```python
from build123d import *

# Parameters (mm, degrees)
SKETCH1_R           = 20
SKETCH1_R_2         = 17.5
BOSS_EXTRUDE1_DEPTH = 20
SKETCH2_R           = 32
SKETCH2_R_2         = 20
BOSS_EXTRUDE2_DEPTH = 3
SKETCH4_W           = 2.75
SKETCH4_H           = 3
CIRPATTERN1_COUNT   = 3
CHAMFER1_SIZE       = 1
SKETCH5_R           = 21.1
SKETCH5_R_2         = 18.5
CUT_EXTRUDE1_DEPTH  = 1.6
FILLET1_R           = 0.25
FILLET2_R           = 0.1
FILLET3_R           = 1


with BuildPart() as part:
    # Sketch1 → Boss-Extrude1 (new body, symmetric)
    with BuildSketch(Plane.XY):
        Circle(SKETCH1_R)
        Circle(SKETCH1_R_2, mode=Mode.SUBTRACT)
    extrude(amount=BOSS_EXTRUDE1_DEPTH, both=True)

    # Chamfer1
    chamfer1_edges = [part.edges().sort_by_distance(p)[0] for p in [
        (-17.5, 0, -20),
    ]]
    chamfer(chamfer1_edges, length=CHAMFER1_SIZE)


with BuildPart() as body_2:
    # Sketch2 → Boss-Extrude2 (new body)
    with BuildSketch(Plane.XY.offset(20)):
        Circle(SKETCH2_R)
        Circle(SKETCH2_R_2, mode=Mode.SUBTRACT)
    extrude(amount=-BOSS_EXTRUDE2_DEPTH)

    # Sketch4 → M5 Clearance Hole1 (revolve, cut)
    with BuildSketch(Plane(origin=(0, 26, 17), x_dir=(0, 1, 0), z_dir=(1, 0, 0))):
        with Locations((1.375, 1.5)):
            Rectangle(SKETCH4_W, SKETCH4_H)
    m5_clearance_hole1 = revolve(axis=Axis((0, 26, 10.65), (0, 0, 1)), mode=Mode.SUBTRACT)

    # CirPattern1: M5 Clearance Hole1 ×3 about axis
    cirpattern1_axis = Axis((0, 0, 0), (0, 0, 1))
    for i in range(1, CIRPATTERN1_COUNT):
        add(m5_clearance_hole1.rotate(cirpattern1_axis, i * 360 / CIRPATTERN1_COUNT), mode=Mode.SUBTRACT)


with BuildPart() as part_1:
    add(part.part)

    # Combine1: union body 2
    add(body_2.part)

    # Sketch5 → Cut-Extrude1 (cut)
    with BuildSketch(Plane.XY.offset(20)):
        Circle(SKETCH5_R)
        Circle(SKETCH5_R_2, mode=Mode.SUBTRACT)
    extrude(amount=-CUT_EXTRUDE1_DEPTH, mode=Mode.SUBTRACT)

    # Fillet1
    fillet1_edges = [part_1.edges().sort_by_distance(p)[0] for p in [
        (-21.1, 0, 18.4),
        (-18.5, 0, 18.4),
    ]]
    fillet(fillet1_edges, radius=FILLET1_R)

    # Fillet2
    fillet2_edges = [part_1.edges().sort_by_distance(p)[0] for p in [
        (-21.1, 0, 20),
        (-18.5, 0, 20),
    ]]
    fillet(fillet2_edges, radius=FILLET2_R)

    # Fillet3
    fillet3_edges = [part_1.edges().sort_by_distance(p)[0] for p in [
        (-20, 0, 17),
    ]]
    fillet(fillet3_edges, radius=FILLET3_R)


solid = part_1.part
```
The listing builds one solid part. Answer for the finished solid, in the listing's coordinates (mm). A direction names the side the tool comes from. Give positions to 0.01 mm unless a question says otherwise; leave off trailing zeros. Order: outer loops, then holes, each group sorted by start corner. A loop starts at its lowest first (then second) coordinate and runs counter-clockwise, first axis right, second up.
1) Find section A-A on x = -22. Write down the section's boundary in (y, z), then the cut area to 3 significant figures.
Reported:
outline: (-23.24, 17) - (-15.7, 17) - (-15.7, 20) - (-23.24, 20) - close; (-10.3, 17) - (23.24, 17) - (23.24, 20) - (-10.3, 20) - close
area: 123 mm2
2) For faces 1 (the face through (20.126, 6.338, 19.284)), 2 (the face through (-4.336, -19.524, -1.748)), 3 (the face through (-19.832, -13.596, 18.521)), determine the directions among +Z, -Z, +X, -X, +Y, -Y from which every point of the face is accessible in a straight line to the end or side of a thin tool.
Reported:
face 1: +Z
face 2: -Z
face 3: +Z, -Z
3) Determine the mould class of faces 4 (the face through (-6.94, -31.24, 18.52)), 5 (the face through (-19, 3, 18.4)), 6 (the face through (6, -18, -20)) for opening direction Y: pulls with the +Y half, pulls with the -Y half, needs draft (parallel to the pull), parting line crosses it, or undercut.
Reported:
face 4: parting line crosses it
face 5: undercut
face 6: needs draft
4) Find section B-B on z = -7. Write down the section's boundary in (x, y), then the cut area to 3 significant figures.
Reported:
outline: circle Ø40 at (0, 0); hole circle Ø35 at (0, 0)
area: 295 mm2
5) Find section D-D on x = 0. Give the number of separate pieces and of enclosed holes in the cut face, then the cut area to 3 significant figures.
Reported:
separate pieces: 3
enclosed holes: 0
area: 247 mm2
6) Find section C-C on y = 26. Write down the section's boundary in (x, z), then the cut area to 3 significant figures.
Reported:
outline: (-18.65, 17) - (-2.75, 17) - (-2.75, 20) - (-18.65, 20) - close; (2.75, 17) - (18.65, 17) - (18.65, 20) - (2.75, 20) - close
area: 95.4 mm2
7) Consider line 1 along X through (y, z) = (-0.5, 11.5); line 2 along Z through (x, y) = (-5, -23); line 3 along X through (y, z) = (-13, 18.15). Determine where each line is inside the solid, lowest interval first.
Reported:
line 1: x = -19.99 to -17.49, 17.49 to 19.99
line 2: z = 17 to 20
line 3: x = -29.24 to -25.27, -19.77 to -11.72, 11.72 to 19.77, 25.27 to 29.24
8) Given P1, Ø3, axis at x = -6.5, z = 4.5, coming from the +Y side; P2, Ø8, axis at y = 14.5, z = 13.5, coming from the -X side; P3, Ø5, axis at x = 0, y = 26, coming from the +Z side (3 decimals); P4, Ø5, axis at x = 12, z = 7.5, coming from the +Y side, each flat-ended and moving along its own axis, determine where each tip first touches the part or whether it passes through.
Reported:
P1: stops at y = 19.36
P2: stops at x = -29.43
P3: passes through
P4: stops at y = 17.6
